Input: part model. Units: mm. Frame: model coordinates. A direction names the side the tool comes from. Round coordinates to 2 decimals unless told otherwise and drop trailing zeros. Order: outer loops, then holes, each group sorted by start corner. A loop starts at its lowest first (then second) coordinate and runs counter-clockwise, first axis right, second up.
Item 1: Mould query, pull axis X, two halves, no side actions, for faces 6 (the flat face through (-3, 15.25, 0)), 7 (the flat face through (14.25, 13, 0)), 8 (the conical face through (5.2, 13.8, -6.8)). Classes: released by +X, released by -X, zero draft, split by the parting line, or undercut.
Item 2: Cut plane B-B on y = -11.75. Output: boundary loops of the cut face in (x, z), then the cut area to 3 significant figures.
Item 3: First-contact query: pin 1 (4 mm diameter, centred on y = -7.5, z = 2.5, fed in from +X); pin 2 (2 mm diameter, centred on x = 11.5, z = -16, fed in from -Y); pin 3 (1.7 mm diameter, centred on x = -11, y = 8, fed in from +Z); pin 4 (4 mm diameter, centred on x = -0.5, z = 12.5, fed in from -Y). Flat tips, straight axial feed; report the tip coordinate or a pass-through.
Item 4: Line query: L1, parallel to Z at x = 7, y = 14.4; L2, parallel to Z at x = -14, y = 11; L3, parallel to X at y = 14.5, z = 7. Output: solid intervals per line, ascending.
Item 5: Cut plane D-D on x = 2. Output: boundary loops of the cut face in (y, z), then the cut area to 3 significant figures.
Item 6: Reachability of faces 1 (the flat face through (-15, -4, -10)), 2 (the conical face through (-8.8, 13.8, -6.8)), 3 (the flat face through (-12, 5.15, 16)), 4 (the cylindrical face through (9.85, 7.12, -15.77)), 5 (the cylindrical face through (-9.43, 6.58, 15.73)) from +Z, -Z, +X, -X, +Y, -Y: full face, straight path, thin tool, end or side. Return the list, or none.
Item 7: Cut plane A-A on x = -11. Output: boundary loops of the cut face in (y, z).
```python
from build123d import *

# Parameters (mm, degrees)
BOSS_EXTRUDE7_DEPTH                            = 17
BOSS_EXTRUDE7_DEPTH_BACK                       = 17
SKETCH1_R                                      = 1.45
SKETCH34_W                                     = 28.4
SKETCH34_H                                     = 7.5
CUT_EXTRUDE11_DEPTH                            = 37.521397837
SKETCH35_R                                     = 5
CUT_EXTRUDE12_DEPTH                            = 25.542055741
CSK_FOR_M3_HEX_SOCKET_COUNTERSUNK_CA_2_COUNT   = 2
CSK_FOR_M3_HEX_SOCKET_COUNTERSUNK_CA_2_PITCH   = 16.5
CSK_FOR_M3_HEX_SOCKET_COUNTERSUNK_CA_3_COUNT   = 2
CSK_FOR_M3_HEX_SOCKET_COUNTERSUNK_CA_3_PITCH   = 18
CSK_FOR_M3_HEX_SOCKET_COUNTERSUNK_CA_4_COUNT   = 2
CSK_FOR_M3_HEX_SOCKET_COUNTERSUNK_CA_4_PITCH   = 24.418230894
FILLET5_R                                      = 1
SKETCH41_W                                     = 28.5
SKETCH41_H                                     = 0.4
CUT_EXTRUDE13_DEPTH                            = 40.895175147
BOSS_EXTRUDE8_START                            = 5
BOSS_EXTRUDE8_DEPTH                            = 5
SKETCH48_R                                     = 1.4
CUT_EXTRUDE14_DEPTH                            = 5
SKETCH49_R                                     = 2.55
CUT_EXTRUDE15_DEPTH                            = 2
SKETCH51_W                                     = 24.851878452
SKETCH51_H                                     = 29.94943361
BOSS_EXTRUDE9_DEPTH                            = 3
CSK_FOR_M3_HEX_SOCKET_COUNTERSUNK_CA_5_A_COUNT = 2
CSK_FOR_M3_HEX_SOCKET_COUNTERSUNK_CA_5_A_PITCH = 14
CSK_FOR_M3_HEX_SOCKET_COUNTERSUNK_CA_6_COUNT   = 2
CSK_FOR_M3_HEX_SOCKET_COUNTERSUNK_CA_6_PITCH   = 19.798989873
CSK_FOR_M3_HEX_SOCKET_COUNTERSUNK_CA_7_COUNT   = 2
CSK_FOR_M3_HEX_SOCKET_COUNTERSUNK_CA_7_PITCH   = 14
SKETCH54_R                                     = 2.55
SKETCH54_W                                     = 20
SKETCH54_H                                     = 16
CUT_EXTRUDE20_DEPTH                            = 2
SKETCH55_W                                     = 29
SKETCH55_H                                     = 7.1
CUT_EXTRUDE21_DEPTH                            = 28.5
SKETCH56_W                                     = 16.7
SKETCH56_H                                     = 5.607195889
CUT_EXTRUDE22_DEPTH                            = 34


with BuildPart() as part:
    # Sketch1 → Boss-Extrude7 (new, two sides: drawn at the far end of the back side and taken through both)
    # profile 1 of 3: a face of its own
    with BuildSketch(Plane.XY.offset(-BOSS_EXTRUDE7_DEPTH_BACK)):
        Polygon((-14.25, 15.25), (-14.25, 11.25), (-8.25, 11.25), (-8.25, 12.25), (8.25, 12.25), (8.25, 11.25), (14.25, 11.25), (14.25, 15.25), align=None)
    # profile 2 of 3: a face of its own
    with BuildSketch(Plane.XY.offset(-BOSS_EXTRUDE7_DEPTH_BACK)):
        with BuildLine():
            Line((14.25, 4.75), (14.25, 11.25))
            Line((14.25, 11.25), (8.25, 11.25))
            Line((8.25, 11.25), (8.25, 8.011710179))
            ThreePointArc((8.25, 8.011710179), (9.502581542, 6.476954843), (10.473180033, 4.75))
            Line((10.473180033, 4.75), (14.25, 4.75))
        make_face()
        with Locations((11, 8)):
            Circle(SKETCH1_R, mode=Mode.SUBTRACT)
    # profile 3 of 3: a face of its own
    with BuildSketch(Plane.XY.offset(-BOSS_EXTRUDE7_DEPTH_BACK)):
        with BuildLine():
            Line((-8.25, 11.25), (-14.25, 11.25))
            Line((-14.25, 11.25), (-14.25, 4.75))
            Line((-14.25, 4.75), (-10.473180033, 4.75))
            ThreePointArc((-10.473180033, 4.75), (-9.502581542, 6.476954843), (-8.25, 8.011710179))
            Line((-8.25, 8.011710179), (-8.25, 11.25))
        make_face()
        with Locations((-11, 8)):
            Circle(SKETCH1_R, mode=Mode.SUBTRACT)
    extrude(amount=BOSS_EXTRUDE7_DEPTH + BOSS_EXTRUDE7_DEPTH_BACK)

    # Sketch34 → Cut-Extrude11 (cut, through all)
    with BuildSketch(Plane.ZY.offset(14.25)):
        with Locations((0, 8.5)):
            Rectangle(SKETCH34_W, SKETCH34_H)
    extrude(amount=-CUT_EXTRUDE11_DEPTH, mode=Mode.SUBTRACT)

    # Sketch35 → Cut-Extrude12 (cut, through all)
    with BuildSketch(Plane(origin=(0, 15.25, 0), x_dir=(1, 0, 0), z_dir=(0, 1, 0))):
        with Locations(Location((0, 0, 0), (0, 0, 270))):
            Circle(SKETCH35_R)
    extrude(amount=-CUT_EXTRUDE12_DEPTH, mode=Mode.SUBTRACT)

    # Sketch40 → CSK for M3 Hex Socket Countersunk Cap Sc (revolve, cut)
    with BuildSketch(Plane(origin=(-8.25, 12.25, 9), x_dir=(0, 0, -1), z_dir=(1, 0, 0))):
        Polygon((0, 0), (0, 3), (1.7, 3), (1.7, 1.66), (3.36, 0), align=None)
    csk_for_m3_hex_socket_countersunk_cap_sc = revolve(axis=Axis((-8.25, 5.9, 9), (0, 1, 0)), mode=Mode.SUBTRACT)

    # CSK for M3 Hex Socket Countersunk Ca 2: CSK for M3 Hex Socket Countersunk Cap Sc ×2
    with Locations(*[(i * CSK_FOR_M3_HEX_SOCKET_COUNTERSUNK_CA_2_PITCH, 0, 0) for i in range(1, CSK_FOR_M3_HEX_SOCKET_COUNTERSUNK_CA_2_COUNT)]):
        add(csk_for_m3_hex_socket_countersunk_cap_sc, mode=Mode.SUBTRACT)

    # CSK for M3 Hex Socket Countersunk Ca 3: CSK for M3 Hex Socket Countersunk Cap Sc ×2
    with Locations(*[(0, 0, -i * CSK_FOR_M3_HEX_SOCKET_COUNTERSUNK_CA_3_PITCH) for i in range(1, CSK_FOR_M3_HEX_SOCKET_COUNTERSUNK_CA_3_COUNT)]):
        add(csk_for_m3_hex_socket_countersunk_cap_sc, mode=Mode.SUBTRACT)

    # CSK for M3 Hex Socket Countersunk Ca 4: CSK for M3 Hex Socket Countersunk Cap Sc ×2
    with Locations(*[Vector(0.6757246285173466, 0, -0.7371541402007413) * (i * CSK_FOR_M3_HEX_SOCKET_COUNTERSUNK_CA_4_PITCH) for i in range(1, CSK_FOR_M3_HEX_SOCKET_COUNTERSUNK_CA_4_COUNT)]):
        add(csk_for_m3_hex_socket_countersunk_cap_sc, mode=Mode.SUBTRACT)

    # Fillet5
    fillet5_edges = [part.edges().sort_by_distance(p)[0] for p in [
        (14.25, 15.25, 0),
        (0, 15.25, -17),
        (0, 15.25, 17),
    ]]
    fillet(fillet5_edges, radius=FILLET5_R)

    # Sketch41 → Cut-Extrude13 (cut, through all)
    with BuildSketch(Plane.XY.offset(17)):
        with Locations((0, 4.95)):
            Rectangle(SKETCH41_W, SKETCH41_H)
    extrude(amount=-CUT_EXTRUDE13_DEPTH, mode=Mode.SUBTRACT)

    # Sketch46 → Boss-Extrude8 (add)
    with BuildSketch(Plane.ZY.offset(14.25).offset(BOSS_EXTRUDE8_START)):
        Polygon((17, -22.75), (17, 5.15), (14.2, 5.15), (14.2, 12.25), (-14.2, 12.25), (-14.2, 5.15), (-17, 5.15), (-17, -22.75), align=None)
        with BuildLine():
            ThreePointArc((-16, 15.25), (-16.707106781, 14.957106781), (-17, 14.25))
            Line((-17, 14.25), (-17, 5.15))
            Line((-17, 5.15), (-14.2, 5.15))
            Line((-14.2, 5.15), (-14.2, 12.25))
            Line((-14.2, 12.25), (14.2, 12.25))
            Line((14.2, 12.25), (14.2, 5.15))
            Line((14.2, 5.15), (17, 5.15))
            Line((17, 5.15), (17, 14.25))
            ThreePointArc((17, 14.25), (16.707106781, 14.957106781), (16, 15.25))
            Line((16, 15.25), (-16, 15.25))
        make_face()
    extrude(amount=-BOSS_EXTRUDE8_DEPTH)

    # Sketch48 → Cut-Extrude14 (cut)
    with BuildSketch(Plane.ZY.offset(19.25)):
        with Locations(Location((-10, -11.75, 0), (0, 0, 270))):
            Circle(SKETCH48_R)
        with Locations(Location((10, -11.75, 0), (0, 0, 270))):
            Circle(SKETCH48_R)
        with Locations(Location((10, 4.25, 0), (0, 0, 270))):
            Circle(SKETCH48_R)
        with Locations(Location((-10, 4.25, 0), (0, 0, 270))):
            Circle(SKETCH48_R)
    extrude(amount=-CUT_EXTRUDE14_DEPTH, mode=Mode.SUBTRACT)

    # Sketch49 → Cut-Extrude15 (cut)
    with BuildSketch(Plane(origin=(-14.25, 0, 0), x_dir=(0, 0, -1), z_dir=(1, 0, 0))):
        with Locations(Location((-10, -11.75, 0), (0, 0, 90))):
            Circle(SKETCH49_R)
        with Locations(Location((10, -11.75, 0), (0, 0, 90))):
            Circle(SKETCH49_R)
        with Locations(Location((10, 4.25, 0), (0, 0, 90))):
            Circle(SKETCH49_R)
        with Locations(Location((-10, 4.25, 0), (0, 0, 90))):
            Circle(SKETCH49_R)
    extrude(amount=-CUT_EXTRUDE15_DEPTH, mode=Mode.SUBTRACT)

    # Sketch51 → Boss-Extrude9 (add)
    with BuildSketch(Plane(origin=(0, 15.25, 0), x_dir=(1, 0, 0), z_dir=(0, 1, 0))):
        Rectangle(SKETCH51_W, SKETCH51_H)
    extrude(amount=-BOSS_EXTRUDE9_DEPTH)

    # Sketch53 → CSK for M3 Hex Socket Countersunk Ca 5 (revolve, cut)
    with BuildSketch(Plane(origin=(-7, 12.25, 7), x_dir=(0, 0, -1), z_dir=(1, 0, 0))):
        Polygon((0, 0), (0, 3), (1.7, 3), (1.7, 1.66), (3.36, 0), align=None)
    csk_for_m3_hex_socket_countersunk_ca_5 = revolve(axis=Axis((-7, 5.9, 7), (0, 1, 0)), mode=Mode.SUBTRACT)

    # CSK for M3 Hex Socket Countersunk Ca 5 a: CSK for M3 Hex Socket Countersunk Ca 5 ×2
    with Locations(*[(0, 0, -i * CSK_FOR_M3_HEX_SOCKET_COUNTERSUNK_CA_5_A_PITCH) for i in range(1, CSK_FOR_M3_HEX_SOCKET_COUNTERSUNK_CA_5_A_COUNT)]):
        add(csk_for_m3_hex_socket_countersunk_ca_5, mode=Mode.SUBTRACT)

    # CSK for M3 Hex Socket Countersunk Ca 6: CSK for M3 Hex Socket Countersunk Ca 5 ×2
    with Locations(*[Vector(0.7071067811865512, 0, -0.7071067811865438) * (i * CSK_FOR_M3_HEX_SOCKET_COUNTERSUNK_CA_6_PITCH) for i in range(1, CSK_FOR_M3_HEX_SOCKET_COUNTERSUNK_CA_6_COUNT)]):
        add(csk_for_m3_hex_socket_countersunk_ca_5, mode=Mode.SUBTRACT)

    # CSK for M3 Hex Socket Countersunk Ca 7: CSK for M3 Hex Socket Countersunk Ca 5 ×2
    with Locations(*[(i * CSK_FOR_M3_HEX_SOCKET_COUNTERSUNK_CA_7_PITCH, 0, 0) for i in range(1, CSK_FOR_M3_HEX_SOCKET_COUNTERSUNK_CA_7_COUNT)]):
        add(csk_for_m3_hex_socket_countersunk_ca_5, mode=Mode.SUBTRACT)

    # Sketch54 → Cut-Extrude20 (cut)
    with BuildSketch(Plane(origin=(-14.25, 0, 0), x_dir=(0, 0, -1), z_dir=(1, 0, 0))):
        with Locations((10, 4.25)):
            Circle(SKETCH54_R)
        with Locations((-10, 4.25)):
            Circle(SKETCH54_R)
        with Locations((-10, -11.75)):
            Circle(SKETCH54_R)
        with Locations((10, -11.75)):
            Circle(SKETCH54_R)
        with Locations((0, -3.75)):
            Rectangle(SKETCH54_W, SKETCH54_H)
        with BuildLine():
            Line((7.45, -11.75), (-7.45, -11.75))
            ThreePointArc((-7.45, -11.75), (-8.196877708, -13.553122292), (-10, -14.3))
            Line((-10, -14.3), (-10, -22.75))
            Line((-10, -22.75), (10, -22.75))
            Line((10, -22.75), (10, -14.3))
            ThreePointArc((10, -14.3), (8.196877708, -13.553122292), (7.45, -11.75))
        make_face()
        with BuildLine():
            Line((-10, 1.7), (-10, 4.25))
            Line((-10, 4.25), (-7.45, 4.25))
            ThreePointArc((-7.45, 4.25), (-11.803122292, 6.053122292), (-10, 1.7))
        make_face()
        with BuildLine():
            Line((-7.45, 4.25), (-10, 4.25))
            Line((-10, 4.25), (-10, 1.7))
            ThreePointArc((-10, 1.7), (-8.196877708, 2.446877708), (-7.45, 4.25))
        make_face()
        with BuildLine():
            ThreePointArc((12.55, 4.25), (10, 6.8), (7.45, 4.25))
            Line((7.45, 4.25), (10, 4.25))
            Line((10, 4.25), (10, 1.7))
            ThreePointArc((10, 1.7), (11.803122292, 2.446877708), (12.55, 4.25))
        make_face()
        with BuildLine():
            Line((10, 4.25), (7.45, 4.25))
            ThreePointArc((7.45, 4.25), (8.196877708, 2.446877708), (10, 1.7))
            Line((10, 1.7), (10, 4.25))
        make_face()
        with BuildLine():
            Line((10, -11.75), (7.45, -11.75))
            ThreePointArc((7.45, -11.75), (8.196877708, -13.553122292), (10, -14.3))
            Line((10, -14.3), (10, -11.75))
        make_face()
        with BuildLine():
            Line((10, -11.75), (10, -9.2))
            ThreePointArc((10, -9.2), (8.196877708, -9.946877708), (7.45, -11.75))
            Line((7.45, -11.75), (10, -11.75))
        make_face()
        with BuildLine():
            Line((-7.45, -11.75), (-10, -11.75))
            Line((-10, -11.75), (-10, -14.3))
            ThreePointArc((-10, -14.3), (-8.196877708, -13.553122292), (-7.45, -11.75))
        make_face()
        with BuildLine():
            ThreePointArc((-7.45, -11.75), (-8.196877708, -9.946877708), (-10, -9.2))
            Line((-10, -9.2), (-10, -11.75))
            Line((-10, -11.75), (-7.45, -11.75))
        make_face()
    extrude(amount=-CUT_EXTRUDE20_DEPTH, mode=Mode.SUBTRACT)

    # Sketch55 → Cut-Extrude21 (cut)
    with BuildSketch(Plane(origin=(14.25, 0, 0), x_dir=(0, 0, -1), z_dir=(1, 0, 0))):
        with Locations((0, 8.7)):
            Rectangle(SKETCH55_W, SKETCH55_H)
    extrude(amount=-CUT_EXTRUDE21_DEPTH, mode=Mode.SUBTRACT)

    # Sketch56 → Cut-Extrude22 (cut)
    with BuildSketch(Plane.XY.offset(17)):
        with Locations((0, 9.462449483)):
            Rectangle(SKETCH56_W, SKETCH56_H)
    extrude(amount=-CUT_EXTRUDE22_DEPTH, mode=Mode.SUBTRACT)


solid = part.part
```
From the geometry:
1. face 6: zero draft
1. face 7: released by +X
1. face 8: undercut
2. outline: (-19.25, -17) - (-14.25, -17) - (-14.25, -12.55) - (-16.25, -12.55) - (-16.25, -11.4) - (-19.25, -11.4) - close; (-19.25, -8.6) - (-16.25, -8.6) - (-16.25, 8.6) - (-19.25, 8.6) - close; (-19.25, 11.4) - (-16.25, 11.4) - (-16.25, 12.55) - (-14.25, 12.55) - (-14.25, 17) - (-19.25, 17) - close
2. area: 103 mm2
3. pin 1: stops at x = -16.25
3. pin 2: stops at y = 5.15
3. pin 3: passes through
3. pin 4: stops at y = 12.27
4. L1: z = -16.99 to -8.7, -5.3 to 5.3, 8.7 to 16.99
4. L2: z = -17 to -14.5, 14.5 to 17
4. L3: x = -19.25 to -8.7, -5.3 to 5.3, 8.7 to 14.22
5. outline: (12.27, -17) - (14.25, -17) arc R1 ccw to (15.25, -16) - (15.25, 16) arc R1 ccw to (14.25, 17) - (12.27, 17) - close
5. area: 101 mm2
6. face 1: +X, -Y
6. face 2: -Y
6. face 3: +Z, -Z, +X, -Y
6. face 4: +Z, -Z
6. face 5: +Z, -Z, -Y
7. outline: (5.15, -17) - (6.55, -17) - (6.55, -14.5) - (5.15, -14.5) - close; (5.15, 14.5) - (6.55, 14.5) - (6.55, 17) - (5.15, 17) - close; (9.45, -17) - (14.25, -17) arc R1 ccw to (15.25, -16) - (15.25, 16) arc R1 ccw to (14.25, 17) - (9.45, 17) - (9.45, 14.5) - (12.25, 14.5) - (12.25, -14.5) - (9.45, -14.5) - close
